```python
from build123d import *

# Parameters (mm, degrees)
SKETCH1_R           = 3.683
SKETCH1_R_2         = 3.4290000000000003
BOSS_EXTRUDE1_DEPTH = 6.35
FILLET1_R           = 2.54
BOSS_EXTRUDE2_DEPTH = 3.8099999999999996
SKETCH3_R           = 3.4290000000000003
CUT_EXTRUDE1_DEPTH  = 12.917885980743574
CUT_EXTRUDE2_DEPTH  = 3.8099999999999996
FILLET2_R           = 2.54


with BuildPart() as part:
    # Sketch1 → Boss-Extrude1 (new body)
    with BuildSketch(Plane(origin=(0, 0, 0), x_dir=(1, 0, 0), z_dir=(0, 1, 0))):
        with Locations(Location((0, 0, 0), (0, 0, 270))):
            Circle(SKETCH1_R)
        with Locations(Location((0, 0, 0), (0, 0, 270))):
            Circle(SKETCH1_R_2, mode=Mode.SUBTRACT)
    extrude(amount=BOSS_EXTRUDE1_DEPTH)

    # Fillet1
    # the kernel refuses this fillet: 2.54 mm, written as the material it takes off along each edge
    with BuildSketch(Plane(origin=(0, 0, 0), x_dir=(-1.8e-16, 0, 1), z_dir=(-1, 0, -1.8e-16))) as fillet1_piece_1:
        with BuildLine():
            CenterArc((5.968999999999999, 1.107160331659332), FILLET1_R, 180, 25.841932763167165)
            Line((3.683, 0), (3.6372799999999996, -0.02214320663318664))
            ThreePointArc((3.6372799999999996, -0.02214320663318664), (3.556, -0.0508), (3.4290000000000003, -0.0508))
            Line((3.4290000000000003, -0.0508), (3.3782, 0))
            Line((3.3782, 0), (3.378199999999999, 1.107160331659332))
            Line((3.378199999999999, 1.107160331659332), (3.4289999999999994, 1.107160331659332))
        make_face()
    revolve(axis=Axis((0, 0, 0), (0, 1, 0)), mode=Mode.SUBTRACT)

    # Sketch2 → Boss-Extrude2 (add)
    with BuildSketch(Plane(origin=(0, 6.35, 0), x_dir=(1, 0, 0), z_dir=(0, 1, 0))):
        Polygon((8.89, 4.762500000000003), (-6.349999999999998, 4.762499999999998), (-6.349999999999998, -4.762500000000002), (8.890000000000002, -4.7624999999999975), align=None)
    extrude(amount=BOSS_EXTRUDE2_DEPTH)

    # Sketch3 → Cut-Extrude1 (cut, through all)
    with BuildSketch(Plane.XZ.offset(-6.35)):
        with Locations(Location((0, 0, 0), (0, 0, 270))):
            Circle(SKETCH3_R)
    extrude(amount=-CUT_EXTRUDE1_DEPTH, mode=Mode.SUBTRACT)

    # Sketch4 → Cut-Extrude2 (cut)
    with BuildSketch(Plane(origin=(0, 10.159999999999998, 0), x_dir=(1, 0, 0), z_dir=(0, 1, 0))):
        Polygon((6.061324865405188, 1.4049999999999996), (6.638675134594815, 1.4049999999999996), (6.927350269189628, 1.9049999999999978), (6.638675134594814, 2.4049999999999994), (6.061324865405189, 2.4049999999999994), (5.772649730810376, 1.9049999999999991), align=None)
        Polygon((7.158290376865474, -1.9049999999999991), (6.754145188432737, -1.2050000000000012), (5.945854811567263, -1.2050000000000012), (5.541709623134526, -1.904999999999999), (5.945854811567265, -2.6049999999999995), (6.754145188432736, -2.6049999999999995), align=None)
    extrude(amount=-CUT_EXTRUDE2_DEPTH, mode=Mode.SUBTRACT)

    # Fillet2
    fillet2_edges = [part.edges().sort_by_distance(p)[0] for p in [
        (-6.349999999999998, 8.254999999999999, -4.762499999999998),
        (-6.349999999999998, 8.254999999999999, 4.762500000000002),
        (8.890000000000002, 8.254999999999999, 4.7624999999999975),
        (8.89, 8.254999999999999, -4.762500000000003),
    ]]
    fillet(fillet2_edges, radius=FILLET2_R)


solid = part.part
```
For this review, take the finished solid that the model builds, in its own axes (mm). A direction names the side the tool comes from. Round coordinates to 2 decimals unless told otherwise and drop trailing zeros. Write each loop counter-clockwise with the first axis right and the second up, starting at its lowest first coordinate (ties: lowest second). Pieces come first, ordered by that corner, then holes.
1) For line 1 along X through (y, z) = (3.1, 0); line 2 along X through (y, z) = (8.75, 0); line 3 along Z through (x, y) = (0, 8.6), list the stretches that pass through material, from the lowest coordinate up.
Answer below:
line 1: x = -3.68 to -3.43, 3.43 to 3.68
line 2: x = -6.35 to -3.43, 3.43 to 8.89
line 3: z = -4.76 to -3.43, 3.43 to 4.76
2) Mouldability with a two-part tool opening along X and no side actions: class faces 3 (the face through (6.4, 8.3, 1.205)), 4 (the face through (8.89, 8, 0)), 5 (the face through (6.3, 8.3, 2.605)), 6 (the face through (-5.586, 8.282, -4.038)) as +X half, -X half, draft (parallel to the pull), parting line (faces both ways), or undercut.
Answer below:
face 3: undercut
face 4: +X half
face 5: undercut
face 6: -X half
3) Take a section at B-B on x = 0. Give the boundary of the cut face in (y, z).
Answer below:
outline: (0, -3.68) - (6.35, -3.68) - (6.35, -4.76) - (10.16, -4.76) - (10.16, -3.43) - (1.11, -3.43) arc R2.54 ccw to start; (0, 3.68) arc R2.54 ccw to (1.11, 3.43) - (10.16, 3.43) - (10.16, 4.76) - (6.35, 4.76) - (6.35, 3.68) - close
4) Take a section at C-C on y = 3. Give the boundary of the cut face in (x, z), then the cut area to 3 significant figures.
Answer below:
outline: circle Ø7.37 at (0, 0); hole circle Ø6.86 at (0, 0)
area: 5.68 mm2
5) Take a section at D-D on z = 4.25. Give the boundary of the cut face in (x, y), then the cut area to 3 significant figures.
Answer below:
outline: (-5.34, 6.35) - (7.88, 6.35) - (7.88, 10.16) - (-5.34, 10.16) - close
area: 50.4 mm2
6) Insertion check: pin 1 Ø1 at (x, y) = (3, 3.5) entering from -Z. The pin has a flat end and moves straight along its axis. Give the tip position at first contact, or say it passes through.
Answer below:
pin 1: stops at z = -2.7
7) Take a section at A-A on z = 0. Give the boundary of the cut face in (x, y), then the cut area to 3 significant figures.
Answer below:
outline: (-6.35, 6.35) - (-3.68, 6.35) - (-3.68, 0) arc R2.54 ccw to (-3.43, 1.11) - (-3.43, 10.16) - (-6.35, 10.16) - close; (3.43, 1.11) arc R2.54 ccw to (3.68, 0) - (3.68, 6.35) - (8.89, 6.35) - (8.89, 10.16) - (3.43, 10.16) - close
area: 35.0 mm2
8) Machinability: for faces 1 (the face through (-3.267, 3.131, 1.699)), 2 (the face through (8.126, 8.282, -4.038)), which of the approach directions +Z, -Z, +X, -X, +Y, -Y give a long, thin tool a straight path to every point of the face, cutting with its end or side? Answer none if there is none.
Answer below:
face 1: -Y
face 2: -Z, +X, +Y, -Y
